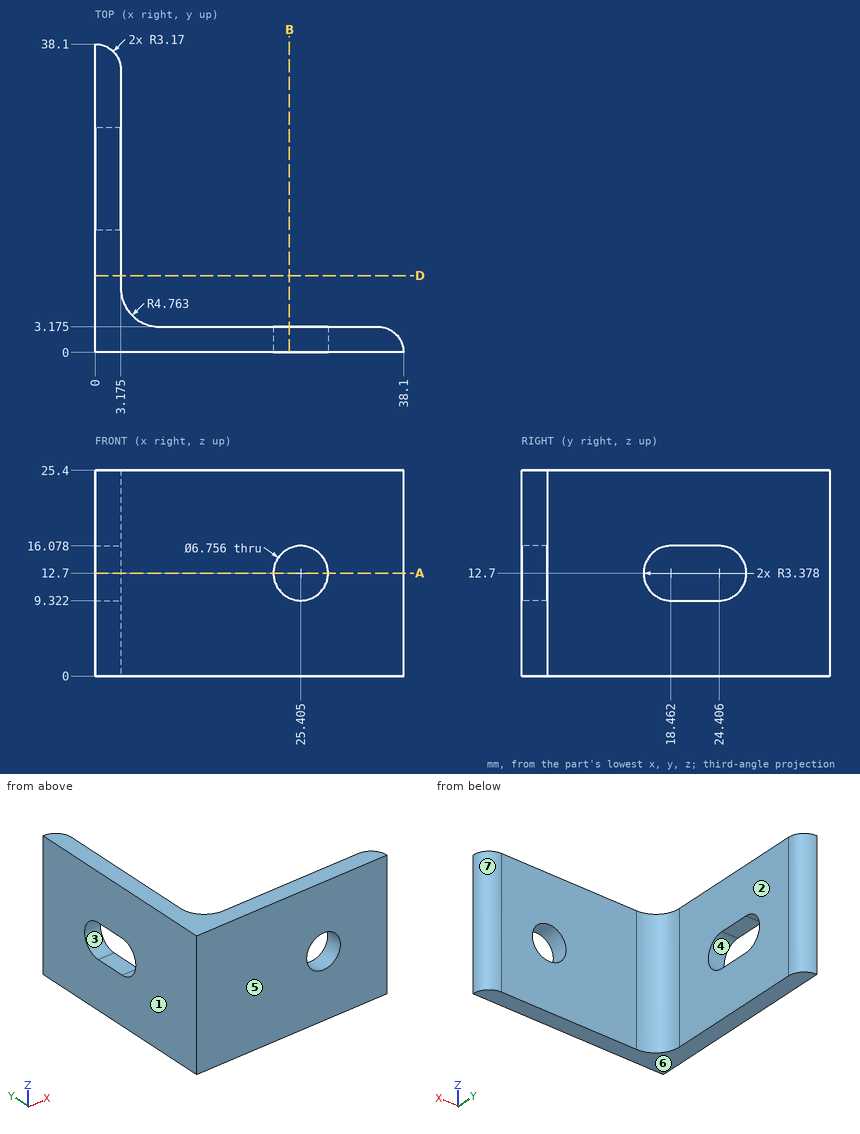
Part print with two shaded views. Sizes in mm from the minimum x, y, z corner. A direction names the side the tool comes from. Round coordinates to 2 decimals unless told otherwise and drop trailing zeros. Write each loop counter-clockwise with the first axis right and the second up, starting at its lowest first coordinate (ties: lowest second). Pieces come first, ordered by that corner, then holes. Notation, with made-up numbers: M -10.5,70.5 L 42.5,70.5 A21 cw 42.5,94.5 Z; hole C 83.5,-7.5 d6. An arc over 180 degrees is marked long. Use CSV: the item, a comma, the result in double quotes.
1. Flat gauge pins, fed straight in: pin 1 (4 mm diameter, centred on y = 16.5, z = 17.5, fed in from +X) (1 decimal); pin 2 (10 mm diameter, centred on x = 27.5, z = 20.5, fed in from +Y) (1 decimal); pin 3 (2.5 mm diameter, centred on x = 2, y = 22, fed in from -Z); pin 4 (6 mm diameter, centred on x = 25.41, z = 12.7, fed in from -Y). Where does each tip first touch, or does it go through?
Reply:
pin 1,"stops at x = 3.2"
pin 2,"stops at y = 3.2"
pin 3,"stops at z = 0"
pin 4,"passes through"
2. Saw through at D-D (y = 9.5). Give the cut face in (x, z) (1 decimal).
Reply:
outline,"M 0,0 L 3.2,0 L 3.2,25.4 L 0,25.4 Z"
3. Two-plate mould, pull along Y, no slides. Class the marked faces 4, 5, 6 and 7: +Y half, -Y half, draft (parallel to the pull), parting line (faces both ways), or undercut.
Reply:
face 4,"undercut"
face 5,"-Y half"
face 6,"draft"
face 7,"+Y half"
4. Saw through at B-B (x = 24). Give the cut face in (y, z) (1 decimal).
Reply:
outline,"M 0,0 L 3.2,0 L 3.2,9.6 L 0,9.6 Z; M 0,15.8 L 3.2,15.8 L 3.2,25.4 L 0,25.4 Z"
5. Saw through at A-A (z = 12.7). State how many separate pieces and enclosed holes the cut face has, plus the area to 3 significant figures.
Reply:
separate pieces,"3"
enclosed holes,"0"
area,"171 mm²"
6. Tool access for the marked faces 1, 2 and 3: list every direction of +Z, -Z, +X, -X, +Y, -Y with a clear straight run to the whole face (end or side of a thin tool).
Reply:
face 1,"+Z, -Z, -X, +Y, -Y"
face 2,"+Z, -Z, +X, +Y"
face 3,"+X, -X"
7. Wall check: probe 1 along Y at (x, z) = (13, 2.25) (1 decimal); probe 2 along X at (y, z) = (2.1, 12.7) (1 decimal); probe 3 along X at (y, z) = (1.2, 12.7) (1 decimal). Give the ranges that are in metal, low to high. Write a range as from..to.
Reply:
probe 1,"y = 0..3.2"
probe 2,"x = 0..22, 28.8..37.3"
probe 3,"x = 0..22, 28.8..37.9"
